For this review, use the dimensioned drawing (mm, ordinates from the lowest corner) and the shaded views. A direction names the side the tool comes from. Round coordinates to 2 decimals unless told otherwise and drop trailing zeros. Loops run counter-clockwise (first coordinate to the right, second up) from the corner with the lowest first, then second, coordinate; pieces in that order, holes last. Notation, with made-up numbers: M -12,14 L 42,14 A23 ccw 42,27 Z; hole C -25,62 d11. An arc over 180 degrees is marked long. Answer as a JSON object with one key per item and string values. Group by question number.
Item 1: Consider section B-B (z = 3.5). Give the boundary of the cut face in (x, y).
Item 2: Tool access review of the marked faces 4, 5 and 6: name each direction out of +Z, -Z, +X, -X, +Y, -Y from which nothing blocks a thin tool from reaching the whole face with its end or side.
Item 3: The part is to be moulded in two halves that separate along Y. For the marked faces 1, 2 and 3, say which applies: +Y half, -Y half, draft (parallel to the pull), parting line (faces both ways), or undercut.
Item 4: To check wall thickness, follow line 1 (Z direction, x = 2.5, y = 5.75); line 2 (Z direction, x = 8.5, y = 1.5); line 3 (Y direction, x = 6.75, z = 10) (1 decimal). State the ranges of each line that lie inside material, in increasing order.
Item 5: Consider section A-A (y = 5). Give the boundary of the cut face in (x, z), and give its area (3 significant figures).
Item 6: Consider section D-D (z = 15.5). Give the boundary of the cut face in (x, y).
Item 7: Insertion check: P1, Ø3, axis at y = 1, z = 28.5, coming from the -X side; P2, Ø4, axis at y = 5, z = 22.5, coming from the +X side; P3, Ø1.5, axis at x = 6.5, z = 9.5, coming from the +Y side (1 decimal). Each pin has a flat end and moves straight along its axis. Give the tip position at first contact, or say it passes through.
Item 8: Consider section C-C (x = 4.75). Give the boundary of the cut face in (y, z), and give its area (3 significant figures).
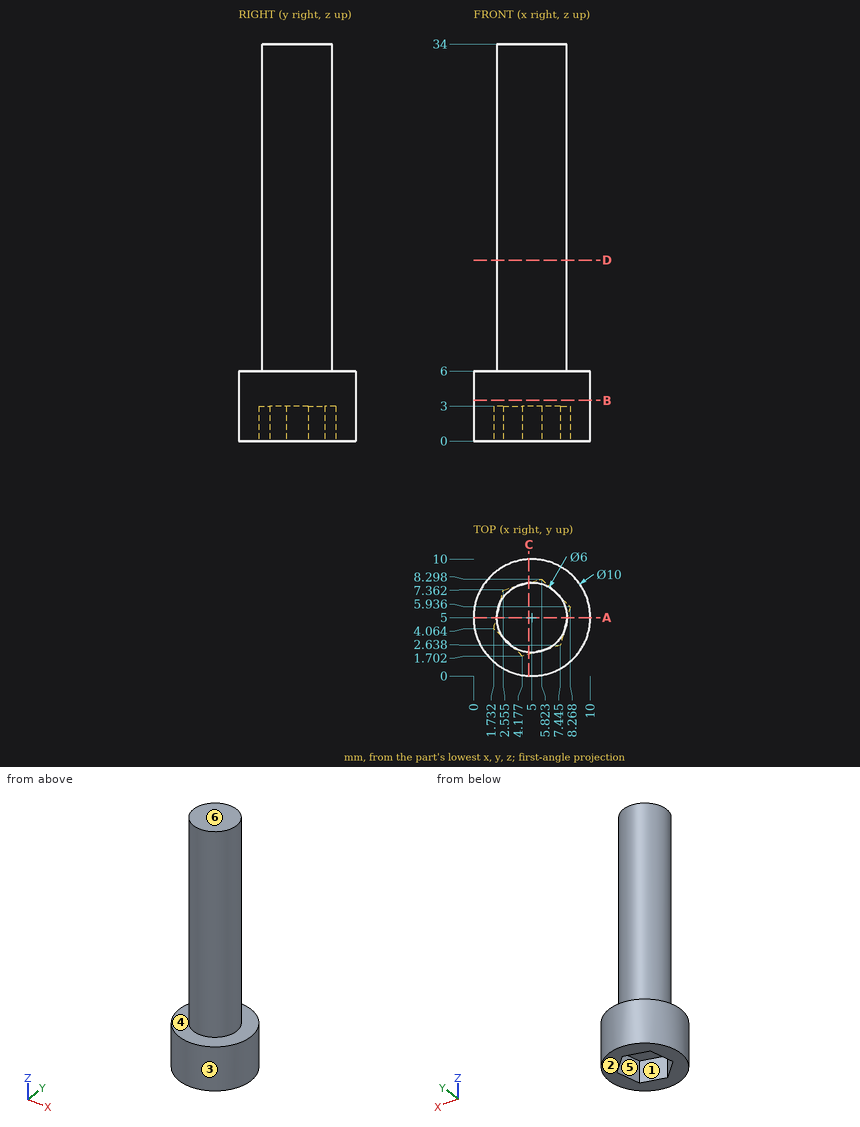
Geometry results:
{
 "1": {"outline": "C 5,5 d10"},
 "2": {"face 4": "+Z", "face 5": "-Z", "face 6": "+Z, +X, -X, +Y, -Y"},
 "3": {"face 1": "undercut", "face 2": "draft", "face 3": "parting line"},
 "4": {"line 1": "z = 3 to 34", "line 2": "z = 0 to 6", "line 3": "y = 2.6 to 7.4"},
 "5": {"outline": "M 0,0 L 1.97,0 L 1.97,3 L 8.03,3 L 8.03,0 L 10,0 L 10,6 L 8,6 L 8,34 L 2,34 L 2,6 L 0,6 Z", "area": "210 mm^2"},
 "6": {"outline": "C 5,5 d6"},
 "7": {"P1": "stops at x = 3.34", "P2": "stops at x = 8", "P3": "stops at y = 7.9"},
 "8": {"outline": "M 0.01,0 L 1.87,0 L 1.87,3 L 7.99,3 L 7.99,0 L 9.99,0 L 9.99,6 L 7.99,6 L 7.99,34 L 2.01,34 L 2.01,6 L 0.01,6 Z", "area": "209 mm^2"}
}
